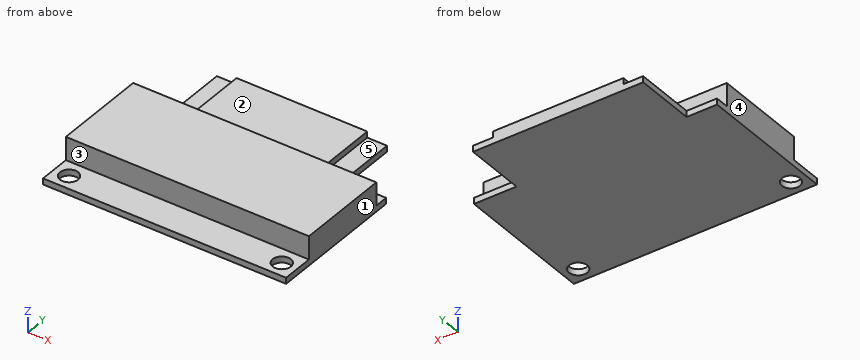
```python
from build123d import *

# Parameters (mm, degrees)
SALIENTE_EXTRUIR1_DEPTH = 1
SALIENTE_EXTRUIR2_DEPTH = 1
CROQUIS3_W              = 40
CROQUIS3_H              = 15.5
SALIENTE_EXTRUIR3_DEPTH = 2.8
CROQUIS4_R              = 1.5
CORTAR_EXTRUIR1_DEPTH   = 1


with BuildPart() as part:
    # Croquis1 → Saliente-Extruir1 (new body)
    with BuildSketch(Plane.XY):
        Polygon((-88.270256069, -7.657514328), (-88.270256069, 15.342485672), (-83.270256069, 15.342485672), (-83.270256069, 25.342485672), (-55.270256069, 25.342485672), (-55.270256069, 15.342485672), (-48.270256069, 15.342485672), (-48.270256069, -7.657514328), align=None)
    extrude(amount=SALIENTE_EXTRUIR1_DEPTH)

    # Croquis2 → Saliente-Extruir2 (add)
    with BuildSketch(Plane.XY.offset(1)):
        Polygon((-88.270256069, -2.407514328), (-88.270256069, 13.092485672), (-80.020256069, 13.092485672), (-80.020256069, 25.342485672), (-58.520256069, 25.342485672), (-58.520256069, 13.092485672), (-48.270256069, 13.092485672), (-48.270256069, -2.407514328), align=None)
    extrude(amount=SALIENTE_EXTRUIR2_DEPTH)

    # Croquis3 → Saliente-Extruir3 (add)
    with BuildSketch(Plane.XY.offset(2)):
        with Locations((-68.270256069, 5.342485672)):
            Rectangle(CROQUIS3_W, CROQUIS3_H)
    extrude(amount=SALIENTE_EXTRUIR3_DEPTH)

    # Croquis4 → Cortar-Extruir1 (cut)
    with BuildSketch(Plane.XY.offset(1)):
        with Locations((-85.770256069, -5.157514328)):
            Circle(CROQUIS4_R)
        with Locations((-50.770256069, -5.157514328)):
            Circle(CROQUIS4_R)
    extrude(amount=-CORTAR_EXTRUIR1_DEPTH, mode=Mode.SUBTRACT)


solid = part.part
```
Geometry: final body of the model. Coordinates: model frame, mm. Face numbers are marked on the shaded views. A direction names the side the tool comes from. Round coordinates to 2 decimals unless told otherwise and drop trailing zeros. Order: outer loops, then holes, each group sorted by start corner. A loop starts at its lowest first (then second) coordinate and runs counter-clockwise, first axis right, second up. Notation, with made-up numbers: (88, -12) -> (147, -12) arc R9 ccw to (147, -5) -> close; hole circle Ø11 at (79, 27). An arc over 180 degrees is marked (long way). Use one line per item in the form item = value.
(1) First-contact query: pin 1 Ø1.1 at (y, z) = (19, 1.5) entering from -X; pin 2 Ø1.1 at (x, z) = (-59.5, 3.5) entering from +Y; pin 3 Ø4 at (x, y) = (-63, -5.5) entering from +Z. Flat tips, straight axial feed; report the tip coordinate or a pass-through.
Results list:
pin_1 = -83.27
pin_2 = 13.09
pin_3 = 1
(2) Section B-B on x = -73. Return loops of the section in (y, z).
Results list:
outline = (-7.66, 0) -> (25.34, 0) -> (25.34, 2) -> (13.09, 2) -> (13.09, 4.8) -> (-2.41, 4.8) -> (-2.41, 1) -> (-7.66, 1) -> close
(3) Section D-D on z = 3.4. Return loops of the section in (x, y), and give its area (3 significant figures).
Results list:
outline = (-88.27, -2.41) -> (-48.27, -2.41) -> (-48.27, 13.09) -> (-88.27, 13.09) -> close
area = 620 mm^2
(4) Ray query, probe 1 along Z at (x, y) = (-66, 18.5); probe 2 along Y at (x, z) = (-84.5, 2.4); probe 3 along Y at (x, z) = (-67, 1.65). Return the intervals inside material, ascending. Write a range as [from, to].
Results list:
probe_1 = [0, 2]
probe_2 = [-2.41, 13.09]
probe_3 = [-2.41, 25.34]
(5) Access query for the marked faces 1, 2, 3, 4 and 5. Directions: +Z, -Z, +X, -X, +Y, -Y. A direction counts if a zero-diameter tool reaches every point of the face in a straight line with its end or side. Return the directions, or none.
Results list:
face_1 = +Z, -Z, +X, +Y, -Y
face_2 = +Z, +X, -X, +Y
face_3 = +Z, +X, -X, -Y
face_4 = +Z, -Z, -X, +Y, -Y
face_5 = +Z, +X, +Y
(6) Section A-A on y = 22. Return loops of the section in (x, z).
Results list:
outline = (-83.27, 0) -> (-55.27, 0) -> (-55.27, 1) -> (-58.52, 1) -> (-58.52, 2) -> (-80.02, 2) -> (-80.02, 1) -> (-83.27, 1) -> close
(7) Section C-C on y = -4.5. Return loops of the section in (x, z).
Results list:
outline = (-88.27, 0) -> (-87.12, 0) -> (-87.12, 1) -> (-88.27, 1) -> close; (-84.42, 0) -> (-52.12, 0) -> (-52.12, 1) -> (-84.42, 1) -> close; (-49.42, 0) -> (-48.27, 0) -> (-48.27, 1) -> (-49.42, 1) -> close
